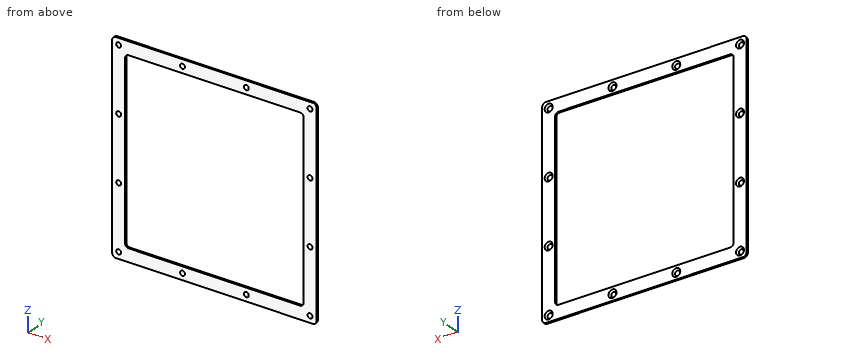
from build123d import *

# Parameters (mm, degrees)
BASE_FLANGE1_DEPTH                            = 1.5875
CUT_EXTRUDE1_DEPTH                            = 255.864612872
CSK_FOR_6_FLAT_HEAD_MACHINE_SCREW1_AT_2_COUNT = 2
CSK_FOR_6_FLAT_HEAD_MACHINE_SCREW1_AT_2_PITCH = 56.261
CSK_FOR_6_FLAT_HEAD_MACHINE_SCREW1_AT_3_COUNT = 2
CSK_FOR_6_FLAT_HEAD_MACHINE_SCREW1_AT_3_PITCH = 177.912903439
CSK_FOR_6_FLAT_HEAD_MACHINE_SCREW1_AT_4_COUNT = 2
CSK_FOR_6_FLAT_HEAD_MACHINE_SCREW1_AT_4_PITCH = 168.783
CSK_FOR_6_FLAT_HEAD_MACHINE_SCREW1_AT_5_COUNT = 2
CSK_FOR_6_FLAT_HEAD_MACHINE_SCREW1_AT_5_PITCH = 112.522
CSK_FOR_6_FLAT_HEAD_MACHINE_SCREW1_AT_6_COUNT = 2
CSK_FOR_6_FLAT_HEAD_MACHINE_SCREW1_AT_6_PITCH = 56.261
CSK_FOR_6_FLAT_HEAD_MACHINE_SCREW1_AT_7_COUNT = 2
CSK_FOR_6_FLAT_HEAD_MACHINE_SCREW1_AT_7_PITCH = 112.522
CSK_FOR_6_FLAT_HEAD_MACHINE_SCREW1_AT_8_COUNT = 2
CSK_FOR_6_FLAT_HEAD_MACHINE_SCREW1_AT_8_PITCH = 168.783
CSK_FOR_6_FLAT_HEAD_MACHINE_SCREW1_AT_9_COUNT = 2
CSK_FOR_6_FLAT_HEAD_MACHINE_SCREW1_AT_9_PITCH = 177.912903439
CSK_FOR_6_FLAT_HEAD_MACHINE_SCREW1_AT_1_COUNT = 2
CSK_FOR_6_FLAT_HEAD_MACHINE_SCREW1_AT_1_PITCH = 202.851920309
CSK_FOR_6_FLAT_HEAD_MACHINE_SCREW1_2_COUNT    = 2
CSK_FOR_6_FLAT_HEAD_MACHINE_SCREW1_2_PITCH    = 202.851920309
CSK_FOR_6_FLAT_HEAD_MACHINE_SCREW1_3_COUNT    = 2
CSK_FOR_6_FLAT_HEAD_MACHINE_SCREW1_3_PITCH    = 238.695207698


# Sheet-metal steps are written as plain solids
with BuildPart() as part:
    # Sketch2 → Base-Flange1 (new body)
    with BuildSketch(Plane(origin=(0, 0, 0), x_dir=(1, 0, 0), z_dir=(0, 1, 0))):
        with BuildLine():
            Line((3.175, 0), (177.038, 0))
            ThreePointArc((177.038, 0), (179.28306403, 0.92993597), (180.213, 3.175))
            Line((180.213, 3.175), (180.213, 177.038))
            ThreePointArc((180.213, 177.038), (179.28306403, 179.28306403), (177.038, 180.213))
            Line((177.038, 180.213), (3.175, 180.213))
            ThreePointArc((3.175, 180.213), (0.92993597, 179.28306403), (0, 177.038))
            Line((0, 177.038), (0, 3.175))
            ThreePointArc((0, 3.175), (0.92993597, 0.92993597), (3.175, 0))
        make_face()
    extrude(amount=-BASE_FLANGE1_DEPTH)

    # Sketch7 → Cut-Extrude1 (cut, through all)
    with BuildSketch(Plane(origin=(0, 0, 0), x_dir=(1, 0, 0), z_dir=(0, 1, 0))):
        with BuildLine():
            Line((14.5288, 168.8592), (165.6842, 168.8592))
            ThreePointArc((165.6842, 168.8592), (167.92926403, 167.92926403), (168.8592, 165.6842))
            Line((168.8592, 165.6842), (168.8592, 14.5288))
            ThreePointArc((168.8592, 14.5288), (167.92926403, 12.28373597), (165.6842, 11.3538))
            Line((165.6842, 11.3538), (14.5288, 11.3538))
            ThreePointArc((14.5288, 11.3538), (12.28373597, 12.28373597), (11.3538, 14.5288))
            Line((11.3538, 14.5288), (11.3538, 165.6842))
            ThreePointArc((11.3538, 165.6842), (12.28373597, 167.92926403), (14.5288, 168.8592))
        make_face()
    extrude(amount=-CUT_EXTRUDE1_DEPTH, mode=Mode.SUBTRACT)

    # Sketch8 → CSK for #6 Flat Head Machine Screw1 (revolve, cut)
    with BuildSketch(Plane(origin=(5.715, 0, -174.4979492), x_dir=(0, 0, 1), z_dir=(1, 0, 0))):
        Polygon((0, 0), (0, 1.5875), (1.8288, 1.5875), (1.8288, 1.972306634), (3.5433, 0), align=None)
    csk_for_6_flat_head_machine_screw1 = revolve(axis=Axis((5.715, 6.35, -174.4979492), (0, -1, 0)), mode=Mode.SUBTRACT)

    # CSK for #6 Flat Head Machine Screw1 at 2: CSK for #6 Flat Head Machine Screw1 ×2
    with Locations(*[(i * CSK_FOR_6_FLAT_HEAD_MACHINE_SCREW1_AT_2_PITCH, 0, 0) for i in range(1, CSK_FOR_6_FLAT_HEAD_MACHINE_SCREW1_AT_2_COUNT)]):
        add(csk_for_6_flat_head_machine_screw1, mode=Mode.SUBTRACT)

    # CSK for #6 Flat Head Machine Screw1 at 3: CSK for #6 Flat Head Machine Screw1 ×2
    with Locations(*[Vector(0.3162277660168381, 0, 0.9486832980505138) * (i * CSK_FOR_6_FLAT_HEAD_MACHINE_SCREW1_AT_3_PITCH) for i in range(1, CSK_FOR_6_FLAT_HEAD_MACHINE_SCREW1_AT_3_COUNT)]):
        add(csk_for_6_flat_head_machine_screw1, mode=Mode.SUBTRACT)

    # CSK for #6 Flat Head Machine Screw1 at 4: CSK for #6 Flat Head Machine Screw1 ×2
    with Locations(*[(0, 0, i * CSK_FOR_6_FLAT_HEAD_MACHINE_SCREW1_AT_4_PITCH) for i in range(1, CSK_FOR_6_FLAT_HEAD_MACHINE_SCREW1_AT_4_COUNT)]):
        add(csk_for_6_flat_head_machine_screw1, mode=Mode.SUBTRACT)

    # CSK for #6 Flat Head Machine Screw1 at 5: CSK for #6 Flat Head Machine Screw1 ×2
    with Locations(*[(0, 0, i * CSK_FOR_6_FLAT_HEAD_MACHINE_SCREW1_AT_5_PITCH) for i in range(1, CSK_FOR_6_FLAT_HEAD_MACHINE_SCREW1_AT_5_COUNT)]):
        add(csk_for_6_flat_head_machine_screw1, mode=Mode.SUBTRACT)

    # CSK for #6 Flat Head Machine Screw1 at 6: CSK for #6 Flat Head Machine Screw1 ×2
    with Locations(*[(0, 0, i * CSK_FOR_6_FLAT_HEAD_MACHINE_SCREW1_AT_6_PITCH) for i in range(1, CSK_FOR_6_FLAT_HEAD_MACHINE_SCREW1_AT_6_COUNT)]):
        add(csk_for_6_flat_head_machine_screw1, mode=Mode.SUBTRACT)

    # CSK for #6 Flat Head Machine Screw1 at 7: CSK for #6 Flat Head Machine Screw1 ×2
    with Locations(*[(i * CSK_FOR_6_FLAT_HEAD_MACHINE_SCREW1_AT_7_PITCH, 0, 0) for i in range(1, CSK_FOR_6_FLAT_HEAD_MACHINE_SCREW1_AT_7_COUNT)]):
        add(csk_for_6_flat_head_machine_screw1, mode=Mode.SUBTRACT)

    # CSK for #6 Flat Head Machine Screw1 at 8: CSK for #6 Flat Head Machine Screw1 ×2
    with Locations(*[(i * CSK_FOR_6_FLAT_HEAD_MACHINE_SCREW1_AT_8_PITCH, 0, 0) for i in range(1, CSK_FOR_6_FLAT_HEAD_MACHINE_SCREW1_AT_8_COUNT)]):
        add(csk_for_6_flat_head_machine_screw1, mode=Mode.SUBTRACT)

    # CSK for #6 Flat Head Machine Screw1 at 9: CSK for #6 Flat Head Machine Screw1 ×2
    with Locations(*[Vector(0.9486832980505139, 0, 0.31622776601683783) * (i * CSK_FOR_6_FLAT_HEAD_MACHINE_SCREW1_AT_9_PITCH) for i in range(1, CSK_FOR_6_FLAT_HEAD_MACHINE_SCREW1_AT_9_COUNT)]):
        add(csk_for_6_flat_head_machine_screw1, mode=Mode.SUBTRACT)

    # CSK for #6 Flat Head Machine Screw1 at 1: CSK for #6 Flat Head Machine Screw1 ×2
    with Locations(*[Vector(0.8320502943378437, 0, 0.5547001962252291) * (i * CSK_FOR_6_FLAT_HEAD_MACHINE_SCREW1_AT_1_PITCH) for i in range(1, CSK_FOR_6_FLAT_HEAD_MACHINE_SCREW1_AT_1_COUNT)]):
        add(csk_for_6_flat_head_machine_screw1, mode=Mode.SUBTRACT)

    # CSK for #6 Flat Head Machine Screw1  2: CSK for #6 Flat Head Machine Screw1 ×2
    with Locations(*[Vector(0.5547001962252293, 0, 0.8320502943378436) * (i * CSK_FOR_6_FLAT_HEAD_MACHINE_SCREW1_2_PITCH) for i in range(1, CSK_FOR_6_FLAT_HEAD_MACHINE_SCREW1_2_COUNT)]):
        add(csk_for_6_flat_head_machine_screw1, mode=Mode.SUBTRACT)

    # CSK for #6 Flat Head Machine Screw1  3: CSK for #6 Flat Head Machine Screw1 ×2
    with Locations(*[Vector(0.7071067811865477, 0, 0.7071067811865475) * (i * CSK_FOR_6_FLAT_HEAD_MACHINE_SCREW1_3_PITCH) for i in range(1, CSK_FOR_6_FLAT_HEAD_MACHINE_SCREW1_3_COUNT)]):
        add(csk_for_6_flat_head_machine_screw1, mode=Mode.SUBTRACT)


solid = part.part
Build history of the part. All positions in model axes, mm. Round coordinates to 2 decimals unless told otherwise and drop trailing zeros. Write each loop counter-clockwise with the first axis right and the second up, starting at its lowest first coordinate (ties: lowest second). Pieces come first, ordered by that corner, then holes. Notation, with made-up numbers: M 32,10 L 43,10 A9 cw 43,22 Z; hole C -17.75,14 d11. An arc over 180 degrees is marked long. Answer as a JSON object with one key per item and string values. Group by question number.
(1) Cut at C-C (y = -0.25). Give the number of separate pieces and of enclosed holes in the cut face, and give its area (3 significant figures).
(2) Cut at A-A (z = -54.5). Give the cut face in (x, y), and give its area (3 significant figures).
(3) Cut at B-B (x = 111.5). Give the cut face in (y, z), and give its area (3 significant figures).
(4) Drill centre lines: L1, parallel to Z at x = 33, y = -0.15; L2, parallel to X at y = -1.4, z = -45.5; L3, parallel to Z at x = 65, y = -0.1. Where is each one in solid material? Low to high.
Responses:
{
 "1": {"separate pieces": "1", "enclosed holes": "13", "area": "7,250 mm2"},
 "2": {"outline": "M 0,-1.59 L 11.35,-1.59 L 11.35,0 L 0,0 Z; M 168.86,-1.59 L 180.21,-1.59 L 180.21,0 L 168.86,0 Z", "area": "36.0 mm2"},
 "3": {"outline": "M -1.59,-180.21 L 0,-180.21 L 0,-168.86 L -1.59,-168.86 Z; M -1.59,-11.35 L 0,-11.35 L 0,0 L -1.59,0 Z", "area": "36.0 mm2"},
 "4": {"L1": "z = -180.21 to -168.86, -11.35 to 0", "L2": "x = 0 to 11.35, 168.86 to 180.21", "L3": "z = -180.21 to -176.17, -172.82 to -168.86, -11.35 to -7.39, -4.04 to 0"}
}
